```python
from build123d import *

# Parameters (mm, degrees)
F0_W     = 0.5
F0_H     = 3.5
F0_R     = 1.25
F1_DEPTH = 6.4
F2_W     = 25.4
F2_H     = 1.4
F2_W_2   = 3.5
F2_H_2   = 1.6
F2_R     = 0.8
F3_DEPTH = 19.8
F4_R     = 0.762


with BuildPart() as f1:
    # F0 (on Top) → F1 (new body)
    with BuildSketch(Plane.XY):
        with Locations((4.1668843009, -11.25)):
            Rectangle(F0_W, F0_H)
        with Locations((-3.3831156991, -11.25)):
            Rectangle(F0_W, F0_H)
        with Locations((-11.9331156991, -11.25)):
            Rectangle(F0_W, F0_H)
        with BuildLine():
            Line((-10.6081156991, 0.7), (-9.8143656991, 0.7))
            Line((-9.8143656991, 0.7), (-9.8143656991, 1.101979753))
            ThreePointArc((-9.8143656991, 1.101979753), (-9.7252470071, 1.317131308), (-9.5100954521, 1.40625))
            Line((-9.5100954521, 1.40625), (6.0168843009, 1.40625))
            Line((6.0168843009, 1.40625), (6.0168843009, 2.2))
            Line((6.0168843009, 2.2), (6.0168843009, 4.6))
            ThreePointArc((6.0168843009, 4.6), (3.6168843009, 7), (1.2168843009, 4.6))
            Line((1.2168843009, 4.6), (1.2168843009, 2.2))
            Line((1.2168843009, 2.2), (-9.5100954521, 2.2))
            ThreePointArc((-9.5100954521, 2.2), (-10.2865130147, 1.8783973155), (-10.6081156991, 1.101979753))
            Line((-10.6081156991, 1.101979753), (-10.6081156991, 0.7))
        make_face()
        with BuildLine():
            Line((6.0168843009, 0), (0, 0))
            Line((0, 0), (-0.7, 0.7))
            Line((-0.7, 0.7), (-5.9126656991, 0.7))
            ThreePointArc((-5.9126656991, 0.7), (-6.5935156991, 1.38085), (-7.2743656991, 0.7))
            Line((-7.2743656991, 0.7), (-9.8143656991, 0.7))
            Line((-9.8143656991, 0.7), (-10.6081156991, 0.7))
            Line((-10.6081156991, 0.7), (-13.7831156991, 0.7))
            Line((-13.7831156991, 0.7), (-13.7831156991, -9.5))
            Line((-13.7831156991, -9.5), (-12.1831156991, -9.5))
            Line((-12.1831156991, -9.5), (-11.6831156991, -9.5))
            Line((-11.6831156991, -9.5), (-3.6331156991, -9.5))
            Line((-3.6331156991, -9.5), (-3.1331156991, -9.5))
            Line((-3.1331156991, -9.5), (3.9168843009, -9.5))
            Line((3.9168843009, -9.5), (4.4168843009, -9.5))
            Line((4.4168843009, -9.5), (6.0168843009, -9.5))
            Line((6.0168843009, -9.5), (6.0168843009, 0))
        make_face()
        with Locations((-8.6831156991, -6.6)):
            Circle(F0_R, mode=Mode.SUBTRACT)
        with Locations((0.8168843009, -6.6)):
            Circle(F0_R, mode=Mode.SUBTRACT)
    extrude(amount=F1_DEPTH)

    # F2 (on face) → F3 (cut, through all)
    with BuildSketch(Plane(origin=(-13.7831156991, 0, 0), x_dir=(0, -1, 0), z_dir=(-1, 0, 0))):
        with Locations((-13.4, 0.7)):
            Rectangle(F2_W, F2_H)
        with Locations((-13.4, 5.7)):
            Rectangle(F2_W, F2_H)
        with Locations((11.25, 0.8)):
            Rectangle(F2_W_2, F2_H_2)
        with Locations((11.25, 5.6)):
            Rectangle(F2_W_2, F2_H_2)
        with Locations((11.25, 3.2)):
            Circle(F2_R)
    extrude(amount=-F3_DEPTH, mode=Mode.SUBTRACT)

    # F4
    f4_edges = [f1.edges().sort_by_distance(p)[0] for p in [
        (-13.783116, -9.5, 3.2),
        (6.016884, 0, 3.2),
        (-13.783116, 0.7, 3.2),
    ]]
    fillet(f4_edges, radius=F4_R)


solid = f1.part
```
For this review, take the finished solid that the model builds, in its own axes (mm). A direction names the side the tool comes from. Coordinates: 2 decimals unless noted, no trailing zeros. Loops run counter-clockwise (first coordinate to the right, second up) from the corner with the lowest first, then second, coordinate; pieces in that order, holes last. Notation, with made-up numbers: (-6, 30.25) - (43, 30.25) arc R23 cw to (43, 40.25) - close; hole circle Ø1 at (-19, 89.25). An arc over 180 degrees is marked (long way). Use one line per item in the form item = value. Start each with the question number.
1) Take a section at C-C (y = -11.25). State the section outline as (x, z) points, plus the area to 3 significant figures.
2) Take a section at A-A (z = 5.5). State the section outline as (x, y) points.
3) To check wall thickness, follow probe 1 along Z at (x, y) = (4.1, -11.25); probe 2 along Y at (x, z) = (4.25, 2.5); probe 3 along Y at (x, z) = (-5, 2.75). State the ranges of each line that lie inside material, in increasing order. Write a range as from..to.
4) Take a section at D-D (x = -9.25). State the section outline as (y, z) points.
5) For pin 1 (1.8 mm diameter, centred on y = -11.25, z = 3.2, fed in from -X); pin 2 (3 mm diameter, centred on x = -6, y = 3, fed in from -Z); pin 3 (5 mm diameter, centred on x = 1.5, y = 4, fed in from +Z), all flat-tipped, find the tip position at first contact; note any pin that passes through.
6) Draft analysis for pull direction Z (two halves, no side actions). For faces 5 (the face through (1.4, 3.2, 1.4)), 6 (the face through (-6.14, 1.21, 3.17)), 7 (the face through (-4, -4, 6.4)), 8 (the face through (4.163, -12.013, 3.44)), state which applies: released by +Z, released by -Z, zero draft, split by the parting line, or undercut.
7) Take a section at B-B (x = -4). State the section outline as (y, z) points, plus the area to 3 significant figures.
8) For faces 1 (the face through (4.417, -12, 2)), 2 (the face through (-4, 2.2, 3)), 3 (the face through (3, 0, 3)), 4 (the face through (-11.683, -12, 2)), list the 3-axis set-ups (+Z, -Z, +X, -X, +Y, -Y) from which the entire face can be reached by the end or side of a thin tool; tool diameter is ignored.
From the geometry:
q1.outline = (-12.18, 1.6) - (-11.68, 1.6) - (-11.68, 2.4) - (-12.18, 2.4) - close; (-12.18, 4) - (-11.68, 4) - (-11.68, 4.8) - (-12.18, 4.8) - close; (-3.63, 1.6) - (-3.13, 1.6) - (-3.13, 2.4) - (-3.63, 2.4) - close; (-3.63, 4) - (-3.13, 4) - (-3.13, 4.8) - (-3.63, 4.8) - close; (3.92, 1.6) - (4.42, 1.6) - (4.42, 2.4) - (3.92, 2.4) - close; (3.92, 4) - (4.42, 4) - (4.42, 4.8) - (3.92, 4.8) - close
q1.area = 2.40 mm2
q2.outline = (-13.78, -8.74) arc R0.76 ccw to (-13.02, -9.5) - (6.02, -9.5) - (6.02, -0.76) arc R0.76 ccw to (5.25, 0) - (0, 0) - (-0.7, 0.7) - (-13.02, 0.7) arc R0.76 ccw to (-13.78, -0.06) - close; hole circle Ø2.5 at (-8.68, -6.6); hole circle Ø2.5 at (0.82, -6.6)
q3.probe_1 = 1.6..2.4, 4..4.8
q3.probe_2 = -13..-11.64, -10.86..0, 1.41..6.91
q3.probe_3 = -9.5..0.7, 1.41..2.2
q4.outline = (-9.5, 0) - (-7.71, 0) - (-7.71, 6.4) - (-9.5, 6.4) - close; (-5.49, 0) - (0.7, 0) - (0.7, 6.4) - (-5.49, 6.4) - close; (1.41, 1.4) - (2.2, 1.4) - (2.2, 5) - (1.41, 5) - close
q5.pin_1 = -12.18
q5.pin_2 = 1.4
q5.pin_3 = 5
q6.face_5 = released by -Z
q6.face_6 = zero draft
q6.face_7 = released by +Z
q6.face_8 = undercut
q7.outline = (-9.5, 0) - (0.7, 0) - (0.7, 6.4) - (-9.5, 6.4) - close; (1.41, 1.4) - (2.2, 1.4) - (2.2, 5) - (1.41, 5) - close
q7.area = 68.1 mm2
q8.face_1 = +Z, -Z, +X, -Y
q8.face_2 = +Z, -Z, -X, +Y
q8.face_3 = +Z, -Z, +X
q8.face_4 = +Z, -Z, -Y
